Geometry check sheet. Reference: the model listing, model coordinates, mm. Face numbers are marked on the shaded views. Coordinates: 2 decimals unless noted, no trailing zeros. Loops run counter-clockwise (first coordinate to the right, second up) from the corner with the lowest first, then second, coordinate; pieces in that order, holes last. Notation, with made-up numbers: (87.5, 75) -> (140.5, 75) arc R30 ccw to (140.5, 101) -> close; hole circle Ø1 at (-8, -22). An arc over 180 degrees is marked (long way). Answer as a JSON object with one key per item and string values.
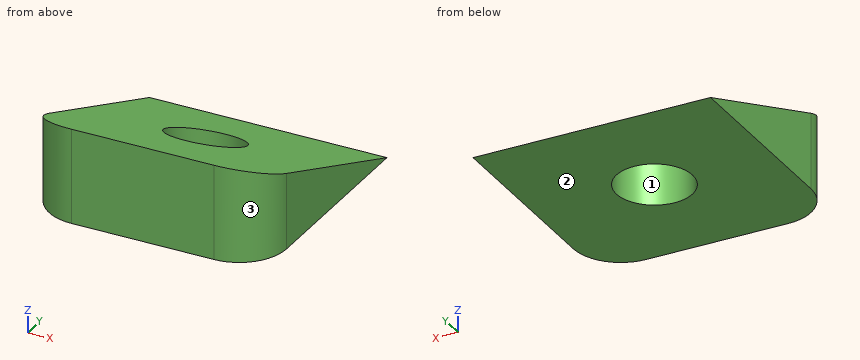
from build123d import *

# Parameters (mm, degrees)
F0_W     = 25
F0_H     = 25
F1_DEPTH = 10
F3_DEPTH = 25
F5_D     = 8
F5_DEPTH = 30
F6_R     = 5


with BuildPart() as f1:
    # F0 (on Top) → F1 (new body)
    with BuildSketch(Plane.XY):
        Rectangle(F0_W, F0_H)
    extrude(amount=F1_DEPTH)

    # F2 (on face) → F3 (cut)
    with BuildSketch(Plane.YZ.offset(12.5)):
        Polygon((12.5, 10), (-12.5, 10), (12.5, 0), align=None)
    extrude(amount=-F3_DEPTH, mode=Mode.SUBTRACT)

    # F5
    with Locations(Plane(origin=(0, 0, 0), x_dir=(1, 0, 0), z_dir=(0, 0, -1))):
        with Locations((0, 0)):
            Hole(F5_D / 2, depth=F5_DEPTH)

    # F6
    f6_edges = [f1.edges().sort_by_distance(p)[0] for p in [
        (12.5, -12.5, 5),
        (-12.5, -12.5, 5),
    ]]
    fillet(f6_edges, radius=F6_R)


solid = f1.part
1. Section check D-D, the plane z = 7. Record the boundary of the cut face in (x, y), then the cut area to 3 significant figures.
Evaluation:
{"outline": "(-12.5, -7.5) arc R5 ccw to (-7.5, -12.5) -> (7.5, -12.5) arc R5 ccw to (12.5, -7.5) -> (12.5, -5) -> (-12.5, -5) -> close", "area": "177 mm^2"}
2. Thickness scan on probe 1 along Y at (x, z) = (0, 1.75) (3 decimals); probe 2 along Y at (x, z) = (0, 4); probe 3 along Z at (x, y) = (-4, -4). Record the ranges inside material, lowest first. Write a range as from..to.
Evaluation:
{"probe 1": "y = -12.5..-4, 4..8.125", "probe 2": "y = -12.5..-4", "probe 3": "z = 0..6.6"}
3. Depth check by flat-ended pin: P1, Ø10, axis at x = 9.5, y = 5, coming from the -Z side; P2, Ø5, axis at x = 8.5, z = 5.5, coming from the +Y side; P3, Ø13, axis at x = 0, y = 0, coming from the +Z side; P4, Ø10, axis at x = -2, y = 1.5, coming from the +Z side. Enter the tip coordinate at first touch or a pass-through.
Evaluation:
{"P1": "stops at z = 0", "P2": "stops at y = 5", "P3": "stops at z = 7.6", "P4": "stops at z = 6.4"}
4. Section check B-B, the plane y = 0. Record the boundary of the cut face in (x, z).
Evaluation:
{"outline": "(-12.5, 0) -> (-4, 0) -> (-4, 5) -> (-12.5, 5) -> close; (4, 0) -> (12.5, 0) -> (12.5, 5) -> (4, 5) -> close"}
5. Section check C-C, the plane z = 2. Record the boundary of the cut face in (x, y).
Evaluation:
{"outline": "(-12.5, -7.5) arc R5 ccw to (-7.5, -12.5) -> (7.5, -12.5) arc R5 ccw to (12.5, -7.5) -> (12.5, 7.5) -> (-12.5, 7.5) -> close; hole circle Ø8 at (0, 0)"}
6. Mould release check, pull along Y, two halves, no side actions. Record for the marked faces 1, 2 and 3: released by +Y, released by -Y, zero draft, split by the parting line, or undercut.
Evaluation:
{"face 1": "undercut", "face 2": "zero draft", "face 3": "released by -Y"}
7. Section check A-A, the plane x = 0. Record the boundary of the cut face in (y, z).
Evaluation:
{"outline": "(-12.5, 0) -> (-4, 0) -> (-4, 6.6) -> (-12.5, 10) -> close; (4, 0) -> (12.5, 0) -> (4, 3.4) -> close"}
